For this review, use the dimensioned drawing (mm, ordinates from the lowest corner) and the shaded views. A direction names the side the tool comes from. Give positions to 0.01 mm unless a question says otherwise; leave off trailing zeros. Write each loop counter-clockwise with the first axis right and the second up, starting at its lowest first coordinate (ties: lowest second). Pieces come first, ordered by that corner, then holes. Notation, with made-up numbers: (44.5, 23) -> (103.5, 23) arc R27 ccw to (103.5, 40) -> close; hole circle Ø10 at (16, 12.25). An arc over 180 degrees is marked (long way). Answer as CSV lines item,"result".
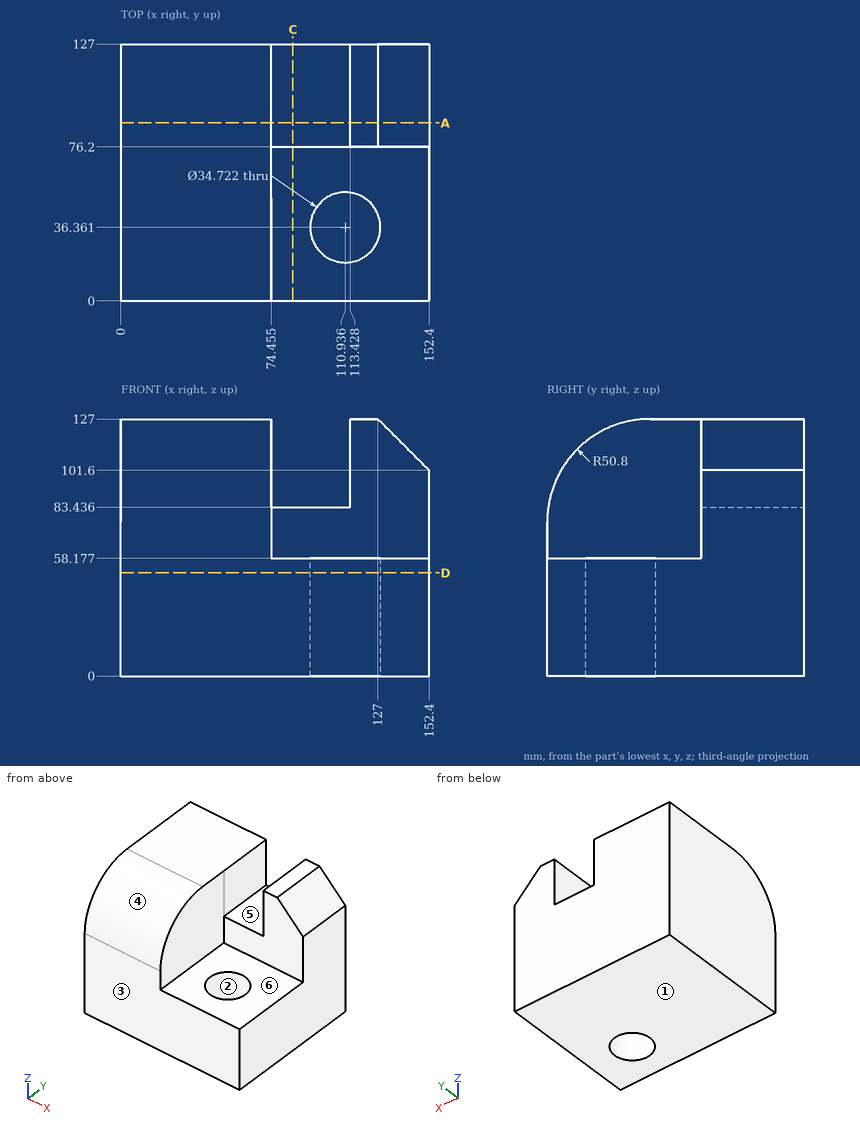
Q1. Add section C-C (x = 85). Write out the cut boundary in (y, z) (1 decimal).
Answer block:
outline,"(0, 0) -> (127, 0) -> (127, 83.4) -> (76.2, 83.4) -> (76.2, 58.2) -> (0, 58.2) -> close"
Q2. Clearance check with flat-ended pins moving along their axes: pin 1 (12 mm diameter, centred on y = 45.5, z = 19.5, fed in from -X); pin 2 (6 mm diameter, centred on x = 81.5, y = 81, fed in from +Z); pin 3 (1 mm diameter, centred on x = 68.5, y = 13.5, fed in from +Z). State where each tip first meets the part, or that it passes through.
Answer block:
pin 1,"stops at x = 0"
pin 2,"stops at z = 83.44"
pin 3,"stops at z = 111.22"
Q3. Add section D-D (z = 51). Write out the cut boundary in (x, y).
Answer block:
outline,"(0, 0) -> (152.4, 0) -> (152.4, 127) -> (0, 127) -> close; hole circle Ø34.72 at (110.94, 36.36)"
Q4. To check wall thickness, follow probe 1 along X at (y, z) = (37.5, 17.5); probe 2 along Z at (x, y) = (76, 44); probe 3 along Z at (x, y) = (102.5, 120.5) (1 decimal). State the ranges of each line that lie inside material, in increasing order. Write a range as [from, to].
Answer block:
probe 1,"x = [0, 93.61], [128.26, 152.4]"
probe 2,"z = [0, 58.18]"
probe 3,"z = [0, 83.4]"
Q5. For the marked faces 4, 5 and 6, list the 3-axis set-ups (+Z, -Z, +X, -X, +Y, -Y) from which the entire face can be reached by the end or side of a thin tool; tool diameter is ignored.
Answer block:
face 4,"+Z, +X, -X, -Y"
face 5,"+Z, +Y, -Y"
face 6,"+Z, +X, -Y"
Q6. Add section A-A (y = 88). Write out the cut boundary in (x, z) (1 decimal).
Answer block:
outline,"(0, 0) -> (152.4, 0) -> (152.4, 101.6) -> (127, 127) -> (113.4, 127) -> (113.4, 83.4) -> (74.5, 83.4) -> (74.5, 127) -> (0, 127) -> close"
Q7. Draft analysis for pull direction Y (two halves, no side actions). For the marked faces 1, 2 and 3, state which applies: released by +Y, released by -Y, zero draft, split by the parting line, or undercut.
Answer block:
face 1,"zero draft"
face 2,"undercut"
face 3,"released by -Y"
